```python
from build123d import *

# Parameters (mm, degrees)
SKETCH_R     = 1.6
PAD_DEPTH    = 20.5
SKETCH001_W  = 10
SKETCH001_H  = 100
POCKET_DEPTH = 1.5
FILLET_R     = 4


with BuildPart() as part:
    # Sketch → Pad (new body)
    with BuildSketch(Plane.XY):
        Polygon((0, 12), (0, 20), (35, 20), (35, 18.5), (8, 18.5), (8, 12), (1.5, 12), (1.5, -12), (8, -12), (8, -18.5), (35, -18.5), (35, -20), (0, -20), (0, -12), align=None)
        with Locations((4, 16)):
            Circle(SKETCH_R, mode=Mode.SUBTRACT)
        with Locations((4, -16)):
            Circle(SKETCH_R, mode=Mode.SUBTRACT)
    extrude(amount=PAD_DEPTH)

    # Sketch001 → Pocket (cut)
    with BuildSketch(Plane.XY):
        with Locations((15, 0)):
            Rectangle(SKETCH001_W, SKETCH001_H)
    extrude(amount=POCKET_DEPTH, mode=Mode.SUBTRACT)

    # Fillet
    fillet_edges = [part.edges().sort_by_distance(p)[0] for p in [
        (0, -20, 10.25),
        (8, -12, 10.25),
        (8, 12, 10.25),
        (0, 20, 10.25),
    ]]
    fillet(fillet_edges, radius=FILLET_R)


solid = part.part
```
Geometry: final body of the model. Coordinates: model frame, mm. A direction names the side the tool comes from. Coordinates: 2 decimals unless noted, no trailing zeros. Loops run counter-clockwise (first coordinate to the right, second up) from the corner with the lowest first, then second, coordinate; pieces in that order, holes last. Notation, with made-up numbers: (-30.75, 53) -> (25.25, 53) arc R36 ccw to (25.25, 89) -> close; hole circle Ø2 at (-1, 21.25). An arc over 180 degrees is marked (long way). Use a Markdown table: item, result. Add a question column.
(1) Section query B-B, the plane z = 19. Return loops of the section in (x, y), plus the area to 3 significant figures.
(2) Mould query, pull axis Y, two halves, no side actions, for faces 1 (the cylindrical face through (1.141, -18.797, 10.394)), 2 (the flat face through (3, 12, 10)), 3 (the flat face through (35, 19, 10)). Classes: pulls with the +Y half, pulls with the -Y half, needs draft (parallel to the pull), parting line crosses it, or undercut.
(3) Section query C-C, the plane y = 17. Return loops of the section in (x, z), plus the area to 3 significant figures.
(4) Section query D-D, the plane y = -1. Return loops of the section in (x, z).
(5) Access query for faces 4 (the cylindrical face through (6.859, -13.203, 10.394)), 5 (the flat face through (20, 19, 1)), 6 (the flat face through (0, 0, 10)). Directions: +Z, -Z, +X, -X, +Y, -Y. A direction counts if a zero-diameter tool reaches every point of the face in a straight line with its end or side. Return the directions, or none.
(6) Line query: line 1 along Y through (x, z) = (30.5, 14); line 2 along Y through (x, z) = (3.5, 5); line 3 along X through (y, z) = (-7, 18.5). Output: solid intervals per line, ascending.
(7) Section query A-A, the plane x = 9.5. Return loops of the section in (y, z).
(8) Pin query (flat end, axial travel): pin 1 Ø0.8 at (y, z) = (-19.5, 1) entering from -X; pin 2 Ø0.8 at (x, y) = (15, 19.5) entering from -Z; pin 3 Ø2 at (y, z) = (-9.5, 5.5) entering from +X. Return the tip coordinate at first contact, or that it passes through.
Answer:
| question | item | result |
|---|---|---|
| 1 | outline | (0, -16) arc R4 ccw to (4, -20) -> (35, -20) -> (35, -18.5) -> (8, -18.5) -> (8, -16) arc R4 ccw to (4, -12) -> (1.5, -12) -> (1.5, 12) -> (4, 12) arc R4 ccw to (8, 16) -> (8, 18.5) -> (35, 18.5) -> (35, 20) -> (4, 20) arc R4 ccw to (0, 16) -> close; hole circle Ø3.2 at (4, -16); hole circle Ø3.2 at (4, 16) |
| 1 | area | 215 mm^2 |
| 2 | face 1 | pulls with the -Y half |
| 2 | face 2 | undercut |
| 2 | face 3 | needs draft |
| 3 | outline | (0.13, 0) -> (2.75, 0) -> (2.75, 20.5) -> (0.13, 20.5) -> close; (5.25, 0) -> (8, 0) -> (8, 20.5) -> (5.25, 20.5) -> close |
| 3 | area | 110 mm^2 |
| 4 | outline | (0, 0) -> (1.5, 0) -> (1.5, 20.5) -> (0, 20.5) -> close |
| 5 | face 4 | +Z, -Z, +X |
| 5 | face 5 | -Z, +Y, -Y |
| 5 | face 6 | +Z, -Z, -X, +Y, -Y |
| 6 | line 1 | y = -20 to -18.5, 18.5 to 20 |
| 6 | line 2 | y = -19.97 to -17.52, -14.48 to -12, 12 to 14.48, 17.52 to 19.97 |
| 6 | line 3 | x = 0 to 1.5 |
| 7 | outline | (-20, 0) -> (-18.5, 0) -> (-18.5, 20.5) -> (-20, 20.5) -> close; (18.5, 0) -> (20, 0) -> (20, 20.5) -> (18.5, 20.5) -> close |
| 8 | pin 1 | stops at x = 1.47 |
| 8 | pin 2 | stops at z = 1.5 |
| 8 | pin 3 | stops at x = 1.5 |
